from build123d import *

# Parameters (mm, degrees)
ESQUISSE1_R              = 37.5
BOSS_EXTRU_1_DEPTH       = 9
ESQUISSE2_R              = 22.5
ENL_V_MAT_EXTRU_1_DEPTH  = 30.5
D_GAGEMENT_M51_OUTLINE_R = 2.9
D_GAGEMENT_M51_DEPTH     = 9


# Read off the part's stored shape, not the designer's step: Dégagement M51
with BuildPart() as part:
    # Esquisse1 → Boss.-Extru.1 (new body)
    with BuildSketch(Plane.XY):
        Circle(ESQUISSE1_R)
    extrude(amount=BOSS_EXTRU_1_DEPTH)

    # Esquisse2 → Enlèv. mat.-Extru.1 (cut)
    with BuildSketch(Plane.XY.offset(9)):
        Circle(ESQUISSE2_R)
    extrude(amount=-ENL_V_MAT_EXTRU_1_DEPTH, mode=Mode.SUBTRACT)

    # Dégagement M51 outline → Dégagement M51 (cut)
    with BuildSketch(Plane.XY):
        with Locations((-15, -25.980762114)):
            Circle(D_GAGEMENT_M51_OUTLINE_R)
        with Locations((-15, 25.980762114)):
            Circle(D_GAGEMENT_M51_OUTLINE_R)
        with Locations((30, 0)):
            Circle(D_GAGEMENT_M51_OUTLINE_R)
    extrude(amount=D_GAGEMENT_M51_DEPTH, mode=Mode.SUBTRACT)


solid = part.part
Input: part model. Units: mm. Frame: model coordinates. Give positions to 0.01 mm unless a question says otherwise; leave off trailing zeros. Order: outer loops, then holes, each group sorted by start corner. A loop starts at its lowest first (then second) coordinate and runs counter-clockwise, first axis right, second up. Notation, with made-up numbers: (82, 25) - (86, 25) arc R19 cw to (86, 51) - close; hole circle Ø3 at (23, 71). An arc over 180 degrees is marked (long way). Answer as a JSON object with one key per item and string values. Group by question number.
Q1. Mould query, pull axis Y, two halves, no side actions, for faces 1 (the face through (32.766, 0.871, 4.437)), 2 (the face through (16.1, -16.1, 9)), 3 (the face through (-4.88, 37.18, 4.44)). Classes: pulls with the +Y half, pulls with the -Y half, needs draft (parallel to the pull), parting line crosses it, or undercut.
Q2. Cut plane A-A, the plane y = 0. Output: boundary loops of the cut face in (x, z), then the cut area to 3 significant figures.
Q3. Cut plane D-D, the plane y = 8.5. Output: boundary loops of the cut face in (x, z), then the cut area to 3 significant figures.
Q4. First-contact query: pin 1 Ø1.5 at (y, z) = (15, 6) entering from -X; pin 2 Ø4 at (y, z) = (16.5, 2.5) entering from +X; pin 3 Ø3 at (y, z) = (30, 5.5) entering from +X. Flat tips, straight axial feed; report the tip coordinate or a pass-through.
Q5. Cut plane C-C, the plane x = -15. Output: boundary loops of the cut face in (y, z), then the cut area to 3 significant figures.
Q6. Cut plane B-B, the plane x = 0. Output: boundary loops of the cut face in (y, z), then the cut area to 3 significant figures.
Q7. Line query: probe 1 along Y at (x, z) = (30, 6); probe 2 along Y at (x, z) = (-16, 6.5); probe 3 along Y at (x, z) = (0, 2.25). Output: solid intervals per line, ascending.
Results:
{
 "1": {"face 1": "undercut", "face 2": "needs draft", "face 3": "parting line crosses it"},
 "2": {"outline": "(-37.5, 0) - (-22.5, 0) - (-22.5, 9) - (-37.5, 9) - close; (22.5, 0) - (27.1, 0) - (27.1, 9) - (22.5, 9) - close; (32.9, 0) - (37.5, 0) - (37.5, 9) - (32.9, 9) - close", "area": "218 mm^2"},
 "3": {"outline": "(-36.52, 0) - (-20.83, 0) - (-20.83, 9) - (-36.52, 9) - close; (20.83, 0) - (36.52, 0) - (36.52, 9) - (20.83, 9) - close", "area": "282 mm^2"},
 "4": {"pin 1": "x = -34.69", "pin 2": "x = 34.58", "pin 3": "x = 24.37"},
 "5": {"outline": "(-34.37, 0) - (-28.88, 0) - (-28.88, 9) - (-34.37, 9) - close; (-23.08, 0) - (-16.77, 0) - (-16.77, 9) - (-23.08, 9) - close; (16.77, 0) - (23.08, 0) - (23.08, 9) - (16.77, 9) - close; (28.88, 0) - (34.37, 0) - (34.37, 9) - (28.88, 9) - close", "area": "212 mm^2"},
 "6": {"outline": "(-37.5, 0) - (-22.5, 0) - (-22.5, 9) - (-37.5, 9) - close; (22.5, 0) - (37.5, 0) - (37.5, 9) - (22.5, 9) - close", "area": "270 mm^2"},
 "7": {"probe 1": "-22.5 to -2.9, 2.9 to 22.5", "probe 2": "-33.92 to -28.7, -23.26 to -15.82, 15.82 to 23.26, 28.7 to 33.92", "probe 3": "-37.5 to -22.5, 22.5 to 37.5"}
}
